from build123d import *

# Parameters (mm, degrees)
F0_W     = 21.1
F0_H     = 87.47
F1_DEPTH = 1.9
F2_W     = 17.6
F2_H     = 83.77
F2_W_2   = 13.6
F2_H_2   = 79.77
F3_DEPTH = 0.8
F4_W     = 9.8
F4_H     = 1.9
F5_DEPTH = 3


with BuildPart() as f1:
    # F0 (on Top) → F1 (new body)
    with BuildSketch(Plane.XY):
        with Locations((10.55, 43.735)):
            Rectangle(F0_W, F0_H)
    extrude(amount=F1_DEPTH)

    # F4 (on face) → F5 (join)
    with BuildSketch(Plane(origin=(0, 0, 0), x_dir=(0, -1, 0), z_dir=(-1, 0, 0))):
        with Locations((-82.57, 0.95)):
            Rectangle(F4_W, F4_H)
    extrude(amount=F5_DEPTH)


with BuildPart() as f3:
    # F2 (on Top) → F3 (new body)
    with BuildSketch(Plane.XY):
        with Locations((36.552641, 44.763047)):
            Rectangle(F2_W, F2_H)
        with Locations((36.552641, 44.763047)):
            Rectangle(F2_W_2, F2_H_2, mode=Mode.SUBTRACT)
    extrude(amount=F3_DEPTH)


solid = f1.part
Part model, mm, in its own coordinate system. A direction names the side the tool comes from. Coordinates: 2 decimals unless noted, no trailing zeros. Loops run counter-clockwise (first coordinate to the right, second up) from the corner with the lowest first, then second, coordinate; pieces in that order, holes last. Notation, with made-up numbers: (64, 86.5) -> (108, 86.5) arc R14 ccw to (108, 109.5) -> close; hole circle Ø9 at (27, 38.5). An arc over 180 degrees is marked (long way). Use a Markdown table: item, result. Add a question column.
Item 1: Band-saw the part on B-B on y = 76.5. Write the cut outline in (x, z).
Item 2: Flat gauge pin, fed straight in: P1, Ø0.6, axis at y = 54.5, z = 0.5, coming from the -X side. Where does the tip first touch, or does it go through?
Item 3: Band-saw the part on A-A on z = 1.6. Write the cut outline in (x, y), plus the area to 3 significant figures.
Item 4: Probe probe 1 along X at (y, z) = (25.5, 0.3); probe 2 along Y at (x, z) = (-1.75, 1.35). List the from-to ranges inside material, lowest first.
Item 5: Which spindle directions (+Z, -Z, +X, -X, +Y, -Y) get a long thin tool onto all of the face, cutting with end or side? Do faces 1 (the flat face through (-1, 77.67, 1)), 2 (the flat face through (9, 44, 1.9)). Say none if no direction does.
Geometry says:
| question | item | result |
|---|---|---|
| 1 | outline | (0, 0) -> (21.1, 0) -> (21.1, 1.9) -> (0, 1.9) -> close |
| 2 | P1 | x = 0 |
| 3 | outline | (-3, 77.67) -> (0, 77.67) -> (0, 0) -> (21.1, 0) -> (21.1, 87.47) -> (-3, 87.47) -> close |
| 3 | area | 1,880 mm² |
| 4 | probe 1 | 0 to 21.1 |
| 4 | probe 2 | 77.67 to 87.47 |
| 5 | face 1 | +Z, -Z, -X, -Y |
| 5 | face 2 | +Z, +X, -X, +Y, -Y |
